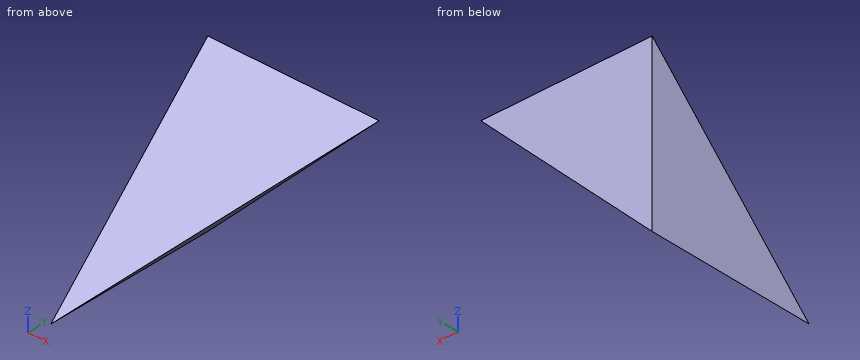
```python
from build123d import *

# Parameters (mm, degrees)
F0_W     = 1000
F0_H     = 1000
F1_DEPTH = 1000
F4_DEPTH = 1000.001
F5_DEPTH = 1000.001


with BuildPart() as f1:
    # F0 (on Top) → F1 (new body)
    with BuildSketch(Plane.XY):
        with Locations((500, 500)):
            Rectangle(F0_W, F0_H)
    extrude(amount=F1_DEPTH)

    # F2 (on face) → F4 (cut, through all)
    with BuildSketch(Plane.YZ.offset(1000)):
        Polygon((0, 0), (1000, 1000), (0, 1000), align=None)
    extrude(amount=-F4_DEPTH, mode=Mode.SUBTRACT)

    # F3 (on face) → F5 (cut, through all)
    with BuildSketch(Plane.XZ):
        Polygon((1000, 0), (1000, 1000), (0, 0), align=None)
    extrude(amount=-F5_DEPTH, mode=Mode.SUBTRACT)


solid = f1.part
```
Part model, mm, in its own coordinate system. Coordinates: 2 decimals unless noted, no trailing zeros. Order: outer loops, then holes, each group sorted by start corner. A loop starts at its lowest first (then second) coordinate and runs counter-clockwise, first axis right, second up. Notation, with made-up numbers: (-38.75, -33) -> (-25.75, -33) arc R23 cw to (-25.75, -18) -> close; hole circle Ø9 at (-26.75, -17). An arc over 180 degrees is marked (long way). Put each result on its own line as item: value. Start each with the question number.
(1) Band-saw the part on D-D (z = 904). Give the cut face in (x, y).
(2) Band-saw the part on C-C (z = 556.5). Give the cut face in (x, y).
(3) Probe line 1 along X through (y, z) = (824, 758.5); line 2 along Z through (x, y) = (363.5, 488.5); line 3 along Y through (x, z) = (152, 895). List the from-to ranges inside material, lowest first. Write a range as [from, to].
(4) Band-saw the part on B-B (x = 277). Give the cut face in (y, z), then the cut area to 3 significant figures.
(5) Band-saw the part on A-A (y = 426.5). Give the cut face in (x, z).
(6) Pin check, flat tips, straight feed: pin 1 Ø8 at (y, z) = (219.5, 123.5) entering from +X; pin 2 Ø1 at (y, z) = (868.5, 709) entering from -X; pin 3 Ø5 at (x, z) = (266.5, 303.5) entering from -Y; pin 4 Ø10 at (x, y) = (670, 815.5) entering from -Z. Stop position of each tip, or through.
Determined:
1. outline: (0, 904) -> (904, 904) -> (904, 1000) -> (0, 1000) -> close
2. outline: (0, 556.5) -> (556.5, 556.5) -> (556.5, 1000) -> (0, 1000) -> close
3. line 1: x = [0, 758.5]
3. line 2: z = [363.5, 488.5]
3. line 3: y = [895, 1000]
4. outline: (277, 277) -> (1000, 277) -> (1000, 1000) -> close
4. area: 261,000 mm²
5. outline: (0, 0) -> (426.5, 426.5) -> (0, 426.5) -> close
6. pin 1: stops at x = 127.5
6. pin 2: stops at x = 0
6. pin 3: stops at y = 301
6. pin 4: stops at z = 665
